```python
from build123d import *

# Parameters (mm, degrees)
F1_W     = 127
F1_H     = 127
F2_DEPTH = 190.5
F3_W     = 127
F3_H     = 127
F4_DEPTH = 127


# Not quite as in the source:
# - a variable given as a bare number and used for a length is read in inches; the dataset says mm whatever the document's units were


with BuildPart() as f2:
    # F1 (on Front) → F2 (new body, symmetric)
    with BuildSketch(Plane.XZ):
        Rectangle(F1_W, F1_H)
    extrude(amount=F2_DEPTH, both=True)

    # F3 (on face) → F4 (join)
    with BuildSketch(Plane.YZ.offset(63.5)):
        with Locations((-127, 0)):
            Rectangle(F3_W, F3_H)
    extrude(amount=F4_DEPTH)


solid = f2.part
```
Part model, mm, in its own coordinate system. A direction names the side the tool comes from. Coordinates: 2 decimals unless noted, no trailing zeros. Write each loop counter-clockwise with the first axis right and the second up, starting at its lowest first coordinate (ties: lowest second). Pieces come first, ordered by that corner, then holes.
Item 1: Pin check, flat tip, straight feed: pin 1 (5 mm diameter, centred on y = 110.5, z = -11.5, fed in from +X). Stop position of the tip, or through.
Item 2: Slice it at A-A (z = -33). Write the cut outline in (x, y).
Item 3: Probe line 1 (Y direction, x = 112.5, z = -34); line 2 (X direction, y = -57, z = 20). List the from-to ranges inside material, lowest first.
Item 4: Which spindle directions (+Z, -Z, +X, -X, +Y, -Y) get a long thin tool onto all of the face, cutting with end or side? Do faces 1 (the face through (63.5, 62, -1)), 2 (the face through (-63.5, -3, -1)). Say none if no direction does.
Item 5: Slice it at C-C (x = 132). Write the cut outline in (y, z).
Item 6: Slice it at B-B (y = -43). Write the cut outline in (x, z).
Results found:
1. pin 1: stops at x = 63.5
2. outline: (-63.5, -190.5) - (190.5, -190.5) - (190.5, -63.5) - (63.5, -63.5) - (63.5, 190.5) - (-63.5, 190.5) - close
3. line 1: y = -190.5 to -63.5
3. line 2: x = -63.5 to 63.5
4. face 1: +Z, -Z, +X, +Y
4. face 2: +Z, -Z, -X, +Y, -Y
5. outline: (-190.5, -63.5) - (-63.5, -63.5) - (-63.5, 63.5) - (-190.5, 63.5) - close
6. outline: (-63.5, -63.5) - (63.5, -63.5) - (63.5, 63.5) - (-63.5, 63.5) - close
